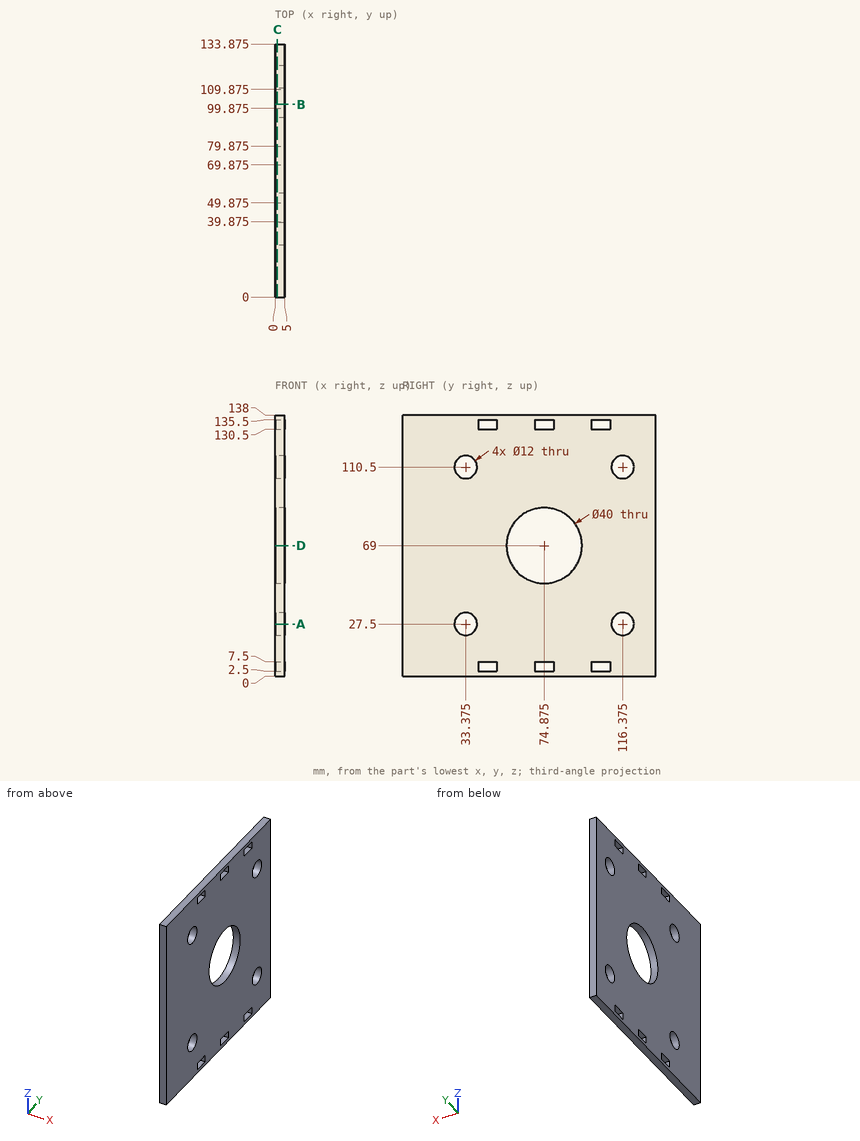
Source: three-view drawing plus pictorial views. Frame: mm from the lowest corner of the part. Give positions to 0.01 mm unless a question says otherwise; leave off trailing zeros. Write each loop counter-clockwise with the first axis right and the second up, starting at its lowest first coordinate (ties: lowest second). Pieces come first, ordered by that corner, then holes. Notation, with made-up numbers: (-34.75, -23.75) -> (14.25, -23.75) arc R8 cw to (14.25, -19.75) -> close; hole circle Ø9 at (14, 10.5). An arc over 180 degrees is marked (long way). Answer in a Markdown table with one row per item.
(1) Section query C-C on x = 1.2. State how many separate pieces and enclosed holes the cut face has, then the cut area to 3 significant figures.
Answers below:
| item | result |
|---|---|
| separate pieces | 1 |
| enclosed holes | 11 |
| area | 16,500 mm^2 |
(2) Section query A-A on z = 27.5. Return loops of the section in (x, y) (1 decimal).
Answers below:
| item | result |
|---|---|
| outline | (0, 0) -> (5, 0) -> (5, 27.4) -> (0, 27.4) -> close; (0, 39.4) -> (5, 39.4) -> (5, 110.4) -> (0, 110.4) -> close; (0, 122.4) -> (5, 122.4) -> (5, 133.9) -> (0, 133.9) -> close |
(3) Ray query, line 1 along Z through (x, y) = (1.9, 101.5); line 2 along Y through (x, z) = (3.35, 27.5) (1 decimal); line 3 along Y through (x, z) = (4.6, 131) (1 decimal). Return the intervals inside material, ascending. Write a range as [from, to].
Answers below:
| item | result |
|---|---|
| line 1 | [0, 2.5], [7.5, 130.5], [135.5, 138] |
| line 2 | [0, 27.4], [39.4, 110.4], [122.4, 133.9] |
| line 3 | [0, 39.9], [49.9, 69.9], [79.9, 99.9], [109.9, 133.9] |
(4) Section query B-B on y = 102. Return loops of the section in (x, z).
Answers below:
| item | result |
|---|---|
| outline | (0, 0) -> (5, 0) -> (5, 2.5) -> (0, 2.5) -> close; (0, 7.5) -> (5, 7.5) -> (5, 130.5) -> (0, 130.5) -> close; (0, 135.5) -> (5, 135.5) -> (5, 138) -> (0, 138) -> close |
(5) Section query D-D on z = 69. Return loops of the section in (x, y) (1 decimal).
Answers below:
| item | result |
|---|---|
| outline | (0, 0) -> (5, 0) -> (5, 54.9) -> (0, 54.9) -> close; (0, 94.9) -> (5, 94.9) -> (5, 133.9) -> (0, 133.9) -> close |
